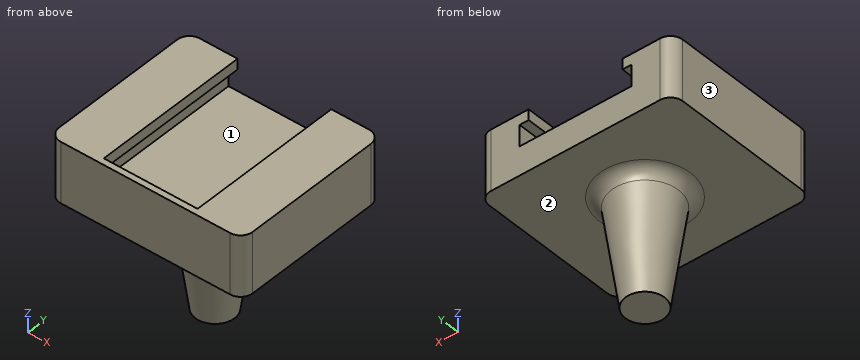
```python
from build123d import *

# Parameters (mm, degrees)
SKETCH1_W           = 32
SKETCH1_H           = 27
BOSS_EXTRUDE1_DEPTH = 10
FILLET1_R           = 2
CUT_EXTRUDE4_DEPTH  = 26
SKETCH4_R           = 5.75
BOSS_EXTRUDE2_DEPTH = 18
BOSS_EXTRUDE2_TAPER = 8
FILLET2_R           = 2


with BuildPart() as part:
    # Sketch1 → Boss-Extrude1 (new body)
    with BuildSketch(Plane.XY):
        Rectangle(SKETCH1_W, SKETCH1_H)
    extrude(amount=BOSS_EXTRUDE1_DEPTH)

    # Fillet1
    fillet1_edges = [part.edges().sort_by_distance(p)[0] for p in [
        (-16, -13.5, 5),
        (16, -13.5, 5),
        (16, 13.5, 5),
        (-16, 13.5, 5),
    ]]
    fillet(fillet1_edges, radius=FILLET1_R)

    # Sketch2 → Cut-Extrude4 (cut)
    with BuildSketch(Plane(origin=(0, 13.5, 0), x_dir=(1, 0, 0), z_dir=(0, 1, 0))):
        Polygon((-7.75, -10), (-7.75, -8.25), (-9.25, -8.25), (-9.25, -4.75), (9.25, -4.75), (9.25, -8.25), (7.75, -8.25), (7.75, -10), align=None)
    extrude(amount=-CUT_EXTRUDE4_DEPTH, mode=Mode.SUBTRACT)

    # Sketch4 → Boss-Extrude2 (add)
    with BuildSketch(Plane(origin=(0, 0, 0), x_dir=(-1, 0, 0), z_dir=(0, 0, -1))):
        Circle(SKETCH4_R)
    extrude(amount=BOSS_EXTRUDE2_DEPTH, taper=BOSS_EXTRUDE2_TAPER)

    # Fillet2
    fillet2_edges = [part.edges().sort_by_distance(p)[0] for p in [
        (5.75, 0, 0),
    ]]
    fillet(fillet2_edges, radius=FILLET2_R)


solid = part.part
```
The listing builds one solid part. Answer for the finished solid, in the listing's coordinates (mm). Face numbers are marked on the shaded views. A direction names the side the tool comes from. Give positions to 0.01 mm unless a question says otherwise; leave off trailing zeros. Order: outer loops, then holes, each group sorted by start corner. A loop starts at its lowest first (then second) coordinate and runs counter-clockwise, first axis right, second up. Notation, with made-up numbers: (4, 74) - (40, 74) arc R28 cw to (40, 105) - close; hole circle Ø7 at (70, 39). An arc over 180 degrees is marked (long way). Use one line per item in the form item = value. Start each with the question number.
(1) Consider line 1 (X direction, y = 10.5, z = 6.25); line 2 (Y direction, x = -6.5, z = 5.25); line 3 (Z direction, x = 10, y = -11.75). Determine where each line is inside the solid, lowest interval first. Write a range as from..to.
(2) For the marked faces 1, 2 and 3, determine the directions among +Z, -Z, +X, -X, +Y, -Y from which every point of the face is accessible in a straight line to the end or side of a thin tool.
(3) A cutting plane is placed at C-C, the plane z = -9. Write down the section's boundary in (x, y).
(4) A cutting plane is placed at D-D, the plane x = 14.5. Write down the section's boundary in (y, z), then the cut area to 3 significant figures.
(5) A cutting plane is placed at A-A, the plane x = 0. Write down the section's boundary in (y, z).
(6) A cutting plane is placed at B-B, the plane x = -12. Write down the section's boundary in (y, z).
(7) Flat-ended cylindrical pins translate along their axes: pin 1 Ø1.6 at (x, y) = (8, -3) entering from -Z; pin 2 Ø4 at (x, y) = (-4, -7.5) entering from -Z; pin 3 Ø6 at (x, z) = (-4, 8) entering from +Y. Find the tip coordinate at first contact, or state that the pin passes through.
Ans:
q1.line_1 = -16..-9.25, 9.25..16
q1.line_2 = -13.5..-12.5
q1.line_3 = 0..10
q2.face_1 = +Y
q2.face_2 = -Z
q2.face_3 = +Z, -Z, -X, +Y, -Y
q3.outline = circle Ø8.97 at (0, 0)
q4.outline = (-13.44, 0) - (13.44, 0) - (13.44, 10) - (-13.44, 10) - close
q4.area = 269 mm^2
q5.outline = (-13.5, 0) - (-7.49, 0) arc R2 cw to (-5.51, -1.72) - (-3.22, -18) - (3.22, -18) - (5.51, -1.72) arc R2 cw to (7.49, 0) - (13.5, 0) - (13.5, 4.75) - (-12.5, 4.75) - (-12.5, 10) - (-13.5, 10) - close
q6.outline = (-13.5, 0) - (13.5, 0) - (13.5, 10) - (-13.5, 10) - close
q7.pin_1 = 0
q7.pin_2 = -0.26
q7.pin_3 = -12.5
